For this review, take the finished solid that the model builds, in its own axes (mm). Face numbers are marked on the shaded views. A direction names the side the tool comes from. Coordinates: 2 decimals unless noted, no trailing zeros. Loops run counter-clockwise (first coordinate to the right, second up) from the corner with the lowest first, then second, coordinate; pieces in that order, holes last. Notation, with made-up numbers: (-34.75, -13.75) -> (-18.75, -13.75) arc R21 ccw to (-18.75, 19.25) -> close; hole circle Ø7 at (-8, -21.5). An arc over 180 degrees is marked (long way). Answer in a Markdown table with one row per item.
from build123d import *

# Parameters (mm, degrees)
BOSS_EXTRU_1_DEPTH           = 10.85
BOSS_EXTRU_1_DEPTH_BACK      = 10.85
BOSS_EXTRU_2_START           = -10.85
ESQUISSE2_W                  = 10
ESQUISSE2_H                  = 7.943097622
BOSS_EXTRU_2_DEPTH           = 4
ESQUISSE3_R                  = 2
ENL_V_MAT_EXTRU_1_DEPTH      = 51.255478557
R_P_TITION_CIRCULAIRE1_COUNT = 2
BOSS_EXTRU_3_DEPTH           = 2
BOSS_EXTRU_3_DEPTH_BACK      = 2
ESQUISSE5_W                  = 55.5
ESQUISSE5_H                  = 16.85
BOSS_EXTRU_4_DEPTH           = 4
CONG_1_R                     = 6
ESQUISSE6_W                  = 63
ESQUISSE6_H                  = 26
BOSS_EXTRU_5_DEPTH           = 4
ESQUISSE7_R                  = 1.6
ENL_V_MAT_EXTRU_2_DEPTH      = 10
CONG_2_START                 = -16
CONG_2_DEPTH                 = 7.9999999


with BuildPart() as part:
    # Esquisse1 → Boss.-Extru.1 (new, two sides: drawn at the far end of the back side and taken through both)
    with BuildSketch(Plane.XY.offset(-BOSS_EXTRU_1_DEPTH_BACK)):
        with BuildLine():
            Line((31.5, 0), (27.75, 0))
            ThreePointArc((27.75, 0), (0, -27.75), (-27.75, 0))
            Line((-27.75, 0), (-31.5, 0))
            ThreePointArc((-31.5, 0), (0, -31.5), (31.5, 0))
        make_face()
    extrude(amount=BOSS_EXTRU_1_DEPTH + BOSS_EXTRU_1_DEPTH_BACK)

    # Esquisse2 → Boss.-Extru.2 (add)
    with BuildSketch(Plane.XY.offset(BOSS_EXTRU_2_START)):
        with Locations((-32.625, 0)):
            Rectangle(ESQUISSE2_W, ESQUISSE2_H)
        with BuildLine():
            ThreePointArc((-33, -2), (-35, 0), (-33, 2))
            Line((-33, 2), (-32.25, 2))
            ThreePointArc((-32.25, 2), (-30.835786438, 1.414213562), (-30.25, 0))
            ThreePointArc((-30.25, 0), (-30.835786438, -1.414213562), (-32.25, -2))
            Line((-32.25, -2), (-33, -2))
        make_face(mode=Mode.SUBTRACT)
    boss_extru_2 = extrude(amount=BOSS_EXTRU_2_DEPTH)

    # Esquisse3 → Enlèv. mat.-Extru.1 (cut, symmetric)
    with BuildSketch(Plane.XY):
        with Locations((-32.25, 0)):
            Circle(ESQUISSE3_R)
    enl_v_mat_extru_1 = extrude(amount=ENL_V_MAT_EXTRU_1_DEPTH, both=True, mode=Mode.SUBTRACT)

    # Répétition circulaire1: Boss.-Extru.2, Enlèv. mat.-Extru.1 ×2 about axis
    r_p_tition_circulaire1_axis = Axis((0, 0, 0), (0, 0, 1))
    add([boss_extru_2.rotate(r_p_tition_circulaire1_axis, i * 360 / R_P_TITION_CIRCULAIRE1_COUNT) for i in range(1, R_P_TITION_CIRCULAIRE1_COUNT)])
    add([enl_v_mat_extru_1.rotate(r_p_tition_circulaire1_axis, i * 360 / R_P_TITION_CIRCULAIRE1_COUNT) for i in range(1, R_P_TITION_CIRCULAIRE1_COUNT)], mode=Mode.SUBTRACT)

    # Esquisse4 → Boss.-Extru.3 (add, two sides: drawn at the far end of the back side and taken through both)
    with BuildSketch(Plane.XY.offset(-BOSS_EXTRU_3_DEPTH_BACK)):
        with BuildLine():
            Line((27.75, -45), (27.75, -3.971548811))
            Line((27.75, -3.971548811), (27.464327773, -3.971548811))
            ThreePointArc((27.464327773, -3.971548811), (0, -27.75), (-27.464327773, -3.971548811))
            Line((-27.464327773, -3.971548811), (-27.75, -3.971548811))
            Line((-27.75, -3.971548811), (-27.75, -45))
            Line((-27.75, -45), (27.75, -45))
        make_face()
    extrude(amount=BOSS_EXTRU_3_DEPTH + BOSS_EXTRU_3_DEPTH_BACK)

    # Esquisse5 → Boss.-Extru.4 (add)
    with BuildSketch(Plane.XZ.offset(45)):
        with Locations((0, -6.425)):
            Rectangle(ESQUISSE5_W, ESQUISSE5_H)
    extrude(amount=BOSS_EXTRU_4_DEPTH)

    # Congé1
    cong_1_edges = [part.edges().sort_by_distance(p)[0] for p in [
        (0, -45, -2),
    ]]
    fillet(cong_1_edges, radius=CONG_1_R)

    # Esquisse6 → Boss.-Extru.5 (add)
    with BuildSketch(Plane(origin=(0, 0, -14.85), x_dir=(-1, 0, 0), z_dir=(0, 0, -1))):
        with Locations((0, -58)):
            Rectangle(ESQUISSE6_W, ESQUISSE6_H)
    extrude(amount=-BOSS_EXTRU_5_DEPTH)

    # Esquisse7 → Enlèv. mat.-Extru.2 (cut)
    with BuildSketch(Plane(origin=(0, 0, -14.85), x_dir=(-1, 0, 0), z_dir=(0, 0, -1))):
        with Locations((-20, -55)):
            Circle(ESQUISSE7_R)
        with Locations((20, -55)):
            Circle(ESQUISSE7_R)
        with Locations((-20, -65)):
            Circle(ESQUISSE7_R)
        with Locations((20, -65)):
            Circle(ESQUISSE7_R)
    extrude(amount=-ENL_V_MAT_EXTRU_2_DEPTH, mode=Mode.SUBTRACT)

    # Congé2: read off the stored shape, not the designer's step
    # Congé2 outline → Congé2 (cut)
    with BuildSketch(Plane.XY.offset(CONG_2_START)):
        with BuildLine():
            Line((-31.5, -71), (-26.5, -71))
            ThreePointArc((-26.5, -71), (-30.035533906, -69.535533906), (-31.5, -66))
            Line((-31.5, -66), (-31.5, -71))
        make_face()
        with BuildLine():
            ThreePointArc((31.5, -66), (30.035533906, -69.535533906), (26.5, -71))
            Line((26.5, -71), (31.5, -71))
            Line((31.5, -71), (31.5, -66))
        make_face()
        with BuildLine():
            Line((-31.5, -45), (-31.5, -50))
            ThreePointArc((-31.5, -50), (-30.035533906, -46.464466094), (-26.5, -45))
            Line((-26.5, -45), (-31.5, -45))
        make_face()
        with BuildLine():
            Line((31.5, -50), (31.5, -45))
            Line((31.5, -45), (26.5, -45))
            ThreePointArc((26.5, -45), (30.035533906, -46.464466094), (31.5, -50))
        make_face()
    extrude(amount=CONG_2_DEPTH, mode=Mode.SUBTRACT)

    # Cong_2 2 outline → Cong_2 2 (revolve, cut)
    with BuildSketch(Plane(origin=(0, -39, -8), x_dir=(0, 1, 0), z_dir=(0, 0, -1))):
        with BuildLine():
            Line((6, -27.75), (6.158770817, -27.75))
            ThreePointArc((6.158770817, -27.75), (6.039851519, -27.130021462), (6, -26.5))
            Line((6, -26.5), (6, -27.75))
        make_face()
        with BuildLine():
            Line((6, 27.75), (6, 26.5))
            ThreePointArc((6, 26.5), (6.039851519, 27.130021462), (6.158770817, 27.75))
            Line((6.158770817, 27.75), (6, 27.75))
        make_face()
    revolve(axis=Axis((0, -39, -8), (1, 0, 0)), mode=Mode.SUBTRACT)


solid = part.part
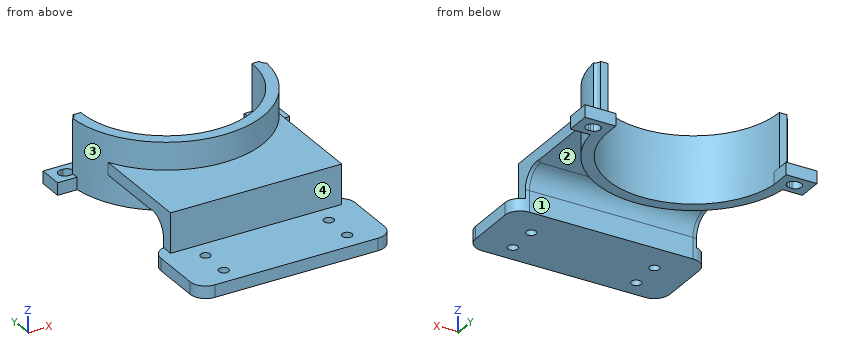
Item 1: Take a section at B-B, the plane x = 0. State the section outline as (y, z) points.
Worked answers:
| item | result |
|---|---|
| outline | (-71, -14.85) -> (-45, -14.85) -> (-45, -8) arc R6 cw to (-39, -2) -> (-31.5, -2) -> (-31.5, -10.85) -> (-27.75, -10.85) -> (-27.75, 10.85) -> (-31.5, 10.85) -> (-31.5, 2) -> (-49, 2) -> (-49, -10.85) -> (-71, -10.85) -> close |
Item 2: Take a section at C-C, the plane y = -24.5. State the section outline as (x, z) points.
Worked answers:
| item | result |
|---|---|
| outline | (-27.75, -2) -> (-19.8, -2) -> (-19.8, -10.85) -> (-13.03, -10.85) -> (-13.03, 10.85) -> (-19.8, 10.85) -> (-19.8, 2) -> (-27.75, 2) -> close; (13.03, -10.85) -> (19.8, -10.85) -> (19.8, -2) -> (27.75, -2) -> (27.75, 2) -> (19.8, 2) -> (19.8, 10.85) -> (13.03, 10.85) -> close |
Item 3: Take a section at D-D, the plane x = -20. State the section outline as (y, z) points, and give its area (3 significant figures).
Worked answers:
| item | result |
|---|---|
| outline | (-71, -14.85) -> (-66.6, -14.85) -> (-66.6, -10.85) -> (-71, -10.85) -> close; (-63.4, -14.85) -> (-56.6, -14.85) -> (-56.6, -10.85) -> (-63.4, -10.85) -> close; (-53.4, -14.85) -> (-45, -14.85) -> (-45, -8) arc R6 cw to (-39, -2) -> (-24.34, -2) -> (-24.34, -10.85) -> (-19.24, -10.85) -> (-19.24, 10.85) -> (-24.34, 10.85) -> (-24.34, 2) -> (-49, 2) -> (-49, -10.85) -> (-53.4, -10.85) -> close |
| area | 331 mm² |
Item 4: Insertion check: pin 1 (1.2 mm diameter, centred on y = -56.5, z = -13.5, fed in from -X); pin 2 (10 mm diameter, centred on x = -7.5, y = -37, fed in from +Z); pin 3 (0.6 mm diameter, centred on x = 32.5, z = -8.5, fed in from -Y). Each pin has a flat end and moves straight along its axis. Give the tip position at first contact, or say it passes through.
Worked answers:
| item | result |
|---|---|
| pin 1 | x = -31.5 |
| pin 2 | z = 2 |
| pin 3 | y = -3.97 |
Item 5: For the marked faces 1, 2, 3 and 4, list the 3-axis set-ups (+Z, -Z, +X, -X, +Y, -Y) from which the entire face can be reached by the end or side of a thin tool; tool diameter is ignored.
Worked answers:
| item | result |
|---|---|
| face 1 | -Z, +X, -X |
| face 2 | -Z |
| face 3 | none |
| face 4 | +Z, +X, -X, -Y |
Item 6: Take a section at A-A, the plane y = -55. State the section outline as (x, z) points.
Worked answers:
| item | result |
|---|---|
| outline | (-31.5, -14.85) -> (-21.6, -14.85) -> (-21.6, -10.85) -> (-31.5, -10.85) -> close; (-18.4, -14.85) -> (18.4, -14.85) -> (18.4, -10.85) -> (-18.4, -10.85) -> close; (21.6, -14.85) -> (31.5, -14.85) -> (31.5, -10.85) -> (21.6, -10.85) -> close |
Item 7: For L1, parallel to X at y = -65, z = -13.9; L2, parallel to Y at x = 20, z = -13.4; L3, parallel to Y at x = 1, z = 2.5, list the stretches that pass through material, from the lowest coordinate up.
Worked answers:
| item | result |
|---|---|
| L1 | -31.5 to -21.6, -18.4 to 18.4, 21.6 to 31.5 |
| L2 | -71 to -66.6, -63.4 to -56.6, -53.4 to -45 |
| L3 | -31.48 to -27.73 |
